Autodesk Inventor part; units mm, degrees
ref_plane "YZ Plane" through (0, 0, 0) normal (1, 0, 0) x (0, 1, 0)
ref_plane "XZ Plane" through (0, 0, 0) normal (0, 1, 0) x (-1, 0, 0)
ref_plane "XY Plane" through (0, 0, 0) normal (0, 0, 1) x (1, 0, 0)
sketch "Sketch2" plane through (0, 0, 0) normal (0, 0, 1) x (1, 0, 0)
  circle A0 centre (0, 0) radius 16.5
  dimension "d0" = 33
extrude "Extrusion1" add sketch "Sketch2" along normal mid plane 12
sketch "Sketch3" plane through (0, 0, 6) normal (0, 0, 1) x (1, 0, 0)
  circle A0 centre (0, 0) radius 1.25
  dimension "d3" = 2.5
extrude "Extrusion2" add sketch "Sketch3" along normal blind 19
ref_plane "Work Plane1" through (0, 0, 15.5) normal (0, 0, 1) x (1, 0, 0)
sketch "Sketch7" plane through (0, 0, 0) normal (0, 0, 1) x (1, 0, 0)
  circle A0 centre (0, 0) radius 21.5
  dimension "d19" = 43
extrude "Extrusion6" add sketch "Sketch7" along normal mid plane 3.7
sketch "Sketch12" plane through (0, 0, -6) normal (0, 0, -1) x (-1, 0, 0)
  circle A0 centre (0, 0) radius 16.5
  circle A1 centre (0, 0) radius 9.5
extrude "Extrusion9" cut sketch "Sketch12" against normal blind 5 contours A1
sketch "Sketch13" plane through (0, 0, -1) normal (0, 0, -1) x (-1, 0, 0)
  circle A0 centre (0, 0) radius 2
  circle A1 centre (0, 0) radius 1.25
  dimension "d33" = 2
extrude "Extrusion10" add sketch "Sketch13" along normal blind 3
fillet "Fillet1" radius 2 1 edges at (9.5, 0, -6)
fillet "Fillet2" radius 2 1 edges at (-16.5, 0, -6)
properties part number "robot" material "PBT Plastic"
Work out the finished part from the listing and answer in its coordinate system (mm). A direction names the side the tool comes from. Round coordinates to 2 decimals unless told otherwise and drop trailing zeros. Write each loop counter-clockwise with the first axis right and the second up, starting at its lowest first coordinate (ties: lowest second). Pieces come first, ordered by that corner, then holes. Notation, with made-up numbers: (14.25, 7.5) -> (47.25, 7.5) arc R20 cw to (47.25, 44.5) -> close; hole circle Ø11 at (-2, 12.25). An arc over 180 degrees is marked (long way). Answer as CSV lines item,"result". Start each with the question number.
(1) Each of these flat-tipped pins is pushed along its axis until it touches: pin 1 (10 mm diameter, centred on x = -7, y = 2, fed in from +Z); pin 2 (1.5 mm diameter, centred on x = -16, y = 1, fed in from -Z); pin 3 (6 mm diameter, centred on x = 6.5, z = -0.5, fed in from -Y). Where does it stop, or does it pass through?
(2) The part is cut by section C-C, the plane z = 0. Give the vertices of the cut face in (x, y).
(3) Find the intervals of material crossed by probe 1 along Y at (x, z) = (0, -2.25); probe 2 along Z at (x, y) = (16.5, 8); probe 3 along Z at (x, y) = (12, 2), in increasing order.
(4) The part is cut by section D-D, the plane x = -17.5. Give the vertices of the cut face in (y, z).
(5) A tool of negligible diameter and unlimited length cuts with its end or side. For faces 1 (the cylindrical face through (0.27, 1.22, -2.48)), 2 (the cylindrical face through (15.24, 6.32, 3.9)), 3 (the flat face through (-9, 8, -6)), from which of +Z, -Z, +X, -X, +Y, -Y can it reach the whole face along a straight path? Write none if from no direction.
(6) The mould has two halves that part along X. Classify faces 4 (the flat face through (0, 0, -1)), 5 (the flat face through (0, 0, 25)), 6 (the cylindrical face through (15.24, -6.32, -2.91)): +X half, -X half, draft (parallel to the pull), parting line (faces both ways), or undercut.
Output values:
1,pin 1,"stops at z = 6"
1,pin 2,"stops at z = -5.84"
1,pin 3,"stops at y = -21.21"
2,outline,"circle Ø43 at (0, 0)"
3,probe 1,"y = -16.5 to -9.5, -2 to -1.25, 1.25 to 2, 9.5 to 16.5"
3,probe 2,"z = -1.85 to 1.85"
3,probe 3,"z = -6 to 6"
4,outline,"(-12.49, -1.85) -> (12.49, -1.85) -> (12.49, 1.85) -> (-12.49, 1.85) -> close"
5,face 1,"-Z"
5,face 2,"+Z"
5,face 3,"-Z, +X, -X, +Y, -Y"
6,face 4,"undercut"
6,face 5,"draft"
6,face 6,"parting line"
